Can you work these out from the model? Positions are in its coordinate system, mm. A direction names the side the tool comes from. Give positions to 0.01 mm unless a question says otherwise; leave off trailing zeros. Write each loop counter-clockwise with the first axis right and the second up, starting at its lowest first coordinate (ties: lowest second). Pieces come first, ordered by that corner, then holes. Notation, with made-up numbers: (17.25, -24.75) - (37.25, -24.75) arc R21 cw to (37.25, 9.25) - close; hole circle Ø5 at (25.5, 74.25). An arc over 180 degrees is marked (long way). Use a Markdown table: item, result. Add a question column.
Autodesk Inventor part; units mm, degrees
ref_plane "YZ Plane" through (0, 0, 0) normal (1, 0, 0) x (0, 1, 0)
ref_plane "XZ Plane" through (0, 0, 0) normal (0, 1, 0) x (-1, 0, 0)
ref_plane "XY Plane" through (0, 0, 0) normal (0, 0, 1) x (1, 0, 0)
sketch "Skizze1" plane through (0, 0, 0) normal (0, 1, 0) x (-1, 0, 0)
  line L0 (9, -4.15) -> (-9, -4.15)
  line L1 (-12, -1.15) -> (-12, 1.15)
  line L2 (-9, 4.15) -> (9, 4.15)
  line L3 (12, 1.15) -> (12, -1.15)
  line L4 (0, -12.6778) -> (0, 8.6418)
  line L5 (13.6706, 0) -> (-20.1804, 0)
  arc A0 (9, -4.15) -> (12, -1.15) centre (9, -1.15) ccw
  arc A1 (12, 1.15) -> (9, 4.15) centre (9, 1.15) ccw
  arc A2 (-9, 4.15) -> (-12, 1.15) centre (-9, 1.15) ccw
  arc A3 (-12, -1.15) -> (-9, -4.15) centre (-9, -1.15) ccw
  point P0 (0, 0)
  point P1 (12, -4.15)
  point P2 (-12, -4.15)
  dimension "d0" = 8.3
  dimension "d1" = 24
  dimension "d2" = 3
extrude "Extrusion1" add sketch "Skizze1" along normal blind 1.6
sketch "Skizze2" plane through (0, 0, 0) normal (0, -1, 0) x (1, 0, 0)
  line L0 (-2.8, 2.5) -> (2.8, 2.5)
  line L1 (2.8, 2.5) -> (2.8, -2.5)
  line L2 (2.8, -2.5) -> (-2.8, -2.5)
  line L3 (-2.8, -2.5) -> (-2.8, 2.5)
  line L4 (-9.3724, 0) -> (8.2101, 0)
  line L5 (0, 7.7773) -> (0, -6.9118)
  point P0 (0, 0)
  dimension "d5" = 5.6
  dimension "d6" = 5
extrude "Extrusion2" add sketch "Skizze2" along normal blind 8.6
sketch "Skizze3" plane through (0, 1.6, 0) normal (0, 1, 0) x (1, 0, 0)
  line L0 (-9, 1.5) -> (-5, 1.5)
  line L1 (-5, 1.5) -> (-5, -1.5)
  line L2 (-5, -1.5) -> (-9, -1.5)
  line L3 (-9, -1.5) -> (-9, 1.5)
  line L4 (-9.8398, 0) -> (1.393, 0)
  line L5 (-12, 1.15) -> (-12, -1.15)
  point P0 (0, 0)
  dimension "d9" = 3
  dimension "d10" = 4
  dimension "d11" = 3
extrude "Extrusion3" add sketch "Skizze3" along normal blind 1
sketch "Skizze4" plane through (0, 2.6, 0) normal (0, 1, 0) x (1, 0, 0)
  circle A0 centre (-7.78, 0) radius 0.65
  line L0 (-5, 1.5) -> (-9, 1.5)
  line L1 (-5, -1.5) -> (-5, 1.5)
  point P0 (0, 0)
  dimension "d14" = 1.3
  dimension "d15" = 1.5
  dimension "d16" = 2.78
extrude "Extrusion4" cut sketch "Skizze4" against normal blind 0.2
properties part number "Mikrofonboard"
Q1. Suppose I cut it at B-B (z = 0). Please give me the cut outline in (x, y).
Q2. Suppose I cut it at A-A (x = 1.25). Please give me the cut outline in (y, z).
Q3. I'm going to push flat-ended pins straight in: P1, Ø0.8, axis at x = -7.5, y = 2.5, coming from the +Z side; P2, Ø1.7, axis at x = -0.5, y = -4.5, coming from the +Z side; P3, Ø3, axis at x = -0.5, y = -5, coming from the -Z side; P4, Ø1, axis at x = -7.5, z = 0.5, coming from the +Y side. Where does each tip first touch, or does it pass through?
Q4. Suppose I cut it at D-D (x = -8.75). Please give me the cut outline in (y, z).
Q5. Suppose I cut it at C-C (y = -6). Please give me the cut outline in (x, z), and give its area (3 significant figures).
Q6. If we mould it in two halves opening along X, with no side actions, what happens to faces 6 (the flat face through (-8, 2.4, 0)), 7 (the flat face through (-7, 2, -1.5)), 8 (the flat face through (-5, 2, 0))? For each: released by +X, released by -X, zero draft, split by the parting line, or undercut.
Q7. On a 3-axis mill with a long thin cutter (end or side, diameter ignored), from which of +Z, -Z, +X, -X, +Y, -Y can I reach the whole of each face in a straight line? I mean faces 1 (the flat face through (-2.8, -4, 0)), 2 (the cylindrical face through (-11.14, 0.79, -3.25)), 3 (the flat face through (-7, 2, 1.5)), 4 (the flat face through (0, -4, -2.5)), 5 (the flat face through (-9, 2, 0)). Say none if no direction works.
Q8. If I drill on probe 1 along Z at (x, y) = (-7.78, 2.5); probe 2 along X at (y, z) = (2.5, 0); probe 3 along Y at (x, z) = (3.75, -1.5), over which ranges is the centre line in solid material (lowest first)? Write a range as [from, to].
Derived:
| question | item | result |
|---|---|---|
| 1 | outline | (-12, 0) - (-2.8, 0) - (-2.8, -8.6) - (2.8, -8.6) - (2.8, 0) - (12, 0) - (12, 1.6) - (-5, 1.6) - (-5, 2.6) - (-7.13, 2.6) - (-7.13, 2.4) - (-8.43, 2.4) - (-8.43, 2.6) - (-9, 2.6) - (-9, 1.6) - (-12, 1.6) - close |
| 2 | outline | (-8.6, -2.5) - (0, -2.5) - (0, -4.15) - (1.6, -4.15) - (1.6, 4.15) - (0, 4.15) - (0, 2.5) - (-8.6, 2.5) - close |
| 3 | P1 | z = 1.5 |
| 3 | P2 | z = 2.5 |
| 3 | P3 | z = -2.5 |
| 3 | P4 | y = 2.6 |
| 4 | outline | (0, -4.15) - (1.6, -4.15) - (1.6, -1.5) - (2.6, -1.5) - (2.6, 1.5) - (1.6, 1.5) - (1.6, 4.15) - (0, 4.15) - close |
| 5 | outline | (-2.8, -2.5) - (2.8, -2.5) - (2.8, 2.5) - (-2.8, 2.5) - close |
| 5 | area | 28.0 mm² |
| 6 | face 6 | undercut |
| 6 | face 7 | zero draft |
| 6 | face 8 | released by +X |
| 7 | face 1 | +Z, -Z, -X, -Y |
| 7 | face 2 | -Z, -X, +Y, -Y |
| 7 | face 3 | +Z, +X, -X, +Y |
| 7 | face 4 | -Z, +X, -X, -Y |
| 7 | face 5 | +Z, -Z, -X, +Y |
| 8 | probe 1 | [-1.5, -0.65], [0.65, 1.5] |
| 8 | probe 2 | [-9, -8.43], [-7.13, -5] |
| 8 | probe 3 | [0, 1.6] |
